from build123d import *

# Parameters (mm, degrees)
BASPROSKE_W         = 6
BASPROSKE_H         = 22
TOOTHCUT_DEPTH      = 32.685959036
TEETHCUTS_COUNT     = 20
TEETHCUTS_ANGLE     = 342
BORSKE_R            = 2
BORE_DEPTH          = 50.0000508
SKETCH1_R           = 5
CUT_EXTRUDE1_DEPTH  = 32.417071791
BOSS_EXTRUDE1_DEPTH = 6
SKETCH3_R           = 3.5
CUT_EXTRUDE2_DEPTH  = 6


with BuildPart() as part:
    # BasProSke → Base-Revolve (revolve)
    with BuildSketch(Plane(origin=(0, 0, 0), x_dir=(1, 0, 0), z_dir=(0, 1, 0)), mode=Mode.PRIVATE) as base_revolve_sk:
        with Locations((3, 11)):
            Rectangle(BASPROSKE_W, BASPROSKE_H)
    revolve(base_revolve_sk.sketch.rotate(Axis((-10, 0, 0), (1, 0, 0)), 180), axis=Axis((-10, 0, 0), (1, 0, 0)))

    # TooCutSke → ToothCut (cut, through all)
    with BuildSketch(Plane(origin=(0, 0, 0), x_dir=(0, 0, -1), z_dir=(1, 0, 0))):
        with BuildLine():
            ThreePointArc((0.986171591, 17.471189616), (0, 17.499), (-0.986171591, 17.471189616))
            ThreePointArc((-0.986171591, 17.471189616), (-1.626916196, 19.798789858), (-2.932850173, 21.829260982))
            ThreePointArc((-2.932850173, 21.829260982), (0, 22.0254), (2.932850173, 21.829260982))
            ThreePointArc((2.932850173, 21.829260982), (1.626916196, 19.798789858), (0.986171591, 17.471189616))
        make_face()
    toothcut = extrude(amount=TOOTHCUT_DEPTH, mode=Mode.SUBTRACT)

    # TeethCuts: ToothCut ×20 about axis
    teethcuts_axis = Axis((-10, 0, 0), (1, 0, 0))
    for i in range(1, TEETHCUTS_COUNT):
        add(toothcut.rotate(teethcuts_axis, i * TEETHCUTS_ANGLE / (TEETHCUTS_COUNT - 1)), mode=Mode.SUBTRACT)

    # BorSke → Bore (cut, symmetric)
    with BuildSketch(Plane(origin=(0, 0, 0), x_dir=(0, 0, -1), z_dir=(1, 0, 0))):
        with Locations(Location((0, 0, 0), (0, 0, 180))):
            Circle(BORSKE_R)
    extrude(amount=BORE_DEPTH, both=True, mode=Mode.SUBTRACT)

    # Sketch1 → Cut-Extrude1 (cut, through all)
    with BuildSketch(Plane(origin=(6, 0, 0), x_dir=(0, 0, -1), z_dir=(1, 0, 0))):
        Circle(SKETCH1_R)
    extrude(amount=-CUT_EXTRUDE1_DEPTH, mode=Mode.SUBTRACT)

    # Sketch2 → Boss-Extrude1 (add)
    with BuildSketch(Plane.ZY):
        with BuildLine():
            Line((-37.617140139, -5), (-8.966472533, -5))
            Line((-8.966472533, -5), (-8.966472533, 5))
            Line((-8.966472533, 5), (-37.617140139, 5))
            ThreePointArc((-37.617140139, 5), (-34.081606234, 3.535533906), (-32.617140139, 0))
            ThreePointArc((-32.617140139, 0), (-34.081606234, -3.535533906), (-37.617140139, -5))
        make_face()
        with BuildLine():
            ThreePointArc((-37.617140139, 5), (-42.617140139, 0), (-37.617140139, -5))
            Line((-37.617140139, -5), (-37.617140139, 5))
        make_face()
        with BuildLine():
            Line((-37.617140139, 5), (-37.617140139, -5))
            ThreePointArc((-37.617140139, -5), (-34.081606234, -3.535533906), (-32.617140139, 0))
            ThreePointArc((-32.617140139, 0), (-34.081606234, 3.535533906), (-37.617140139, 5))
        make_face()
    extrude(amount=-BOSS_EXTRUDE1_DEPTH)

    # Sketch3 → Cut-Extrude2 (cut)
    with BuildSketch(Plane.ZY):
        with Locations((-37.617140139, 0)):
            Circle(SKETCH3_R)
    extrude(amount=-CUT_EXTRUDE2_DEPTH, mode=Mode.SUBTRACT)


solid = part.part
Read the model definition and answer for the solid it produces. Units are mm, in the model's axes. A direction names the side the tool comes from. Give positions to 0.01 mm unless a question says otherwise; leave off trailing zeros. Write each loop counter-clockwise with the first axis right and the second up, starting at its lowest first coordinate (ties: lowest second). Pieces come first, ordered by that corner, then holes. Notation, with made-up numbers: (70, 57) - (75, 57) arc R20 cw to (75, 63) - close; hole circle Ø3 at (80, -28). An arc over 180 degrees is marked (long way). Use CSV: the item, a comma, the result in double quotes. Start each with the question number.
(1) Consider line 1 along Y through (x, z) = (1.35, -37.5); line 2 along Y through (x, z) = (3.7, -7); line 3 along Z through (x, y) = (0.8, 14.5). Determine where each line is inside the solid, lowest interval first.
(2) Given P1, Ø1.5, axis at x = 4.5, y = -10, coming from the -Z side; P2, Ø3, axis at x = 2, z = -22.5, coming from the +Y side; P3, Ø1, axis at x = 3.5, y = 1.5, coming from the +Z side, each flat-ended and moving along its own axis, determine where each tip first touches the part or whether it passes through.
(3) Find section B-B (z = 0). Give the vertices of the cut face in (x, y), plus the area to 3 significant figures.
(4) Find section D-D (z = -22.5). Give the vertices of the cut face in (x, y).
(5) Find section C-C (x = 1.5). Count the separate pieces of the cut face and the enclosed holes in it, plus the area to 3 significant figures.
(6) Determine the mould class of faces 6 (the cylindrical face through (2.958, -10.325, 16.992)), 7 (the flat face through (3, 5, -27)), 8 (the cylindrical face through (2.958, 12.911, -15.037)) for opening direction Z: +Z half, -Z half, draft (parallel to the pull), parting line (faces both ways), or undercut.
(7) Find section A-A (y = 0). Give the vertices of the cut face in (x, z), plus the area to 3 significant figures.
(8) For faces 1 (the flat face through (6, 5, -3)), 2 (the cylindrical face through (2.96, -4.57, 19.35)), 3 (the cylindrical face through (2.958, 0.11, -42.616)), 4 (the cylindrical face through (2.958, -1.607, 19.754)), 5 (the cylindrical face through (2.96, -15.07, 12.97)), determine the directions among +Z, -Z, +X, -X, +Y, -Y from which every point of the face is accessible in a straight line to the end or side of a thin tool.
Findings below:
1,line 1,"-5 to -3.5, 3.5 to 5"
1,line 2,"-17.48 to 17.48"
1,line 3,"-15.75 to -12.11, -9.8 to 9.8, 12.11 to 15.75"
2,P1,"z = -19.84"
2,P2,"y = 5"
2,P3,"z = 20.53"
3,outline,"(0, -17.5) - (6, -17.5) - (6, -5) - (0, -5) - close; (0, 5) - (6, 5) - (6, 17.5) - (0, 17.5) - close"
3,area,"150 mm2"
4,outline,"(0, -5) - (6, -5) - (6, 5) - (0, 5) - close"
5,separate pieces,"1"
5,enclosed holes,"2"
5,area,"1,310 mm2"
6,face 6,"undercut"
6,face 7,"draft"
6,face 8,"-Z half"
7,outline,"(0, -42.62) - (6, -42.62) - (6, -41.12) - (0, -41.12) - close; (0, -34.12) - (6, -34.12) - (6, -5) - (0, -5) - close; (0, 5) - (6, 5) - (6, 17.5) - (0, 17.5) - close"
7,area,"259 mm2"
8,face 1,"+Z, -Z, +X, +Y, -Y"
8,face 2,"+X, -X"
8,face 3,"-Z, +X, -X"
8,face 4,"+Z, +X, -X"
8,face 5,"+X, -X, -Y"
